Could you check a few things on this model? Use its own coordinates, in mm. Give positions to 0.01 mm unless a question says otherwise; leave off trailing zeros. Order: outer loops, then holes, each group sorted by start corner. A loop starts at its lowest first (then second) coordinate and runs counter-clockwise, first axis right, second up. Notation, with made-up numbers: (50.25, -39) - (97.25, -39) arc R16 ccw to (97.25, -10) - close; hole circle Ø10 at (22, 75.5). An arc over 180 degrees is marked (long way). Put each result on its own line as item: value.
from build123d import *

# Parameters (mm, degrees)
CYLINDER002_R     = 0.3
CYLINDER002_DEPTH = 5
CYLINDER001_R     = 1.3
CYLINDER001_DEPTH = 5
CYLINDER_R        = 6
CYLINDER_DEPTH    = 9.5
CYLINDER003_R     = 0.3
CYLINDER003_DEPTH = 5
FUSION_ROLL_ANGLE = -90


with BuildPart() as obj1:
    # Cylinder002 → Cylinder002 (new body)
    with BuildSketch(Plane(origin=(0, -3.8, -5), x_dir=(1, 0, 0), z_dir=(0, 0, 1))):
        Circle(CYLINDER002_R)
    extrude(amount=CYLINDER002_DEPTH)


with BuildPart() as obj2:
    # Cylinder001 → Cylinder001 (new body)
    with BuildSketch(Plane.XY.offset(4.5)):
        Circle(CYLINDER001_R)
    extrude(amount=CYLINDER001_DEPTH)


with BuildPart() as cut:
    # Cylinder → Cylinder (new body)
    with BuildSketch(Plane.XY):
        Circle(CYLINDER_R)
    extrude(amount=CYLINDER_DEPTH)

    # Cut: cut obj2
    add(obj2.part, mode=Mode.SUBTRACT)


with BuildPart() as buzzer12mm:
    # Cylinder003 → Cylinder003 (new body)
    with BuildSketch(Plane(origin=(0, 3.8, -5), x_dir=(1, 0, 0), z_dir=(0, 0, 1))):
        Circle(CYLINDER003_R)
    extrude(amount=CYLINDER003_DEPTH)

    # Fusion: union obj1, Cut
    add(obj1.part)
    add(cut.part)


with BuildPart() as buzzer12mm_1:
    # Fusion roll: moved
    add(buzzer12mm.part.rotate(Axis((0, 0, 0), (1, 0, 0)), FUSION_ROLL_ANGLE))


with BuildPart() as buzzer12mm_2:
    # Fusion placement: moved
    add(buzzer12mm_1.part.moved(Location((33.37, 5.4, -21.62))))


solid = buzzer12mm_2.part
1) I'm going to push flat-ended pins straight in: pin 1 (5 mm diameter, centred on y = 6.5, z = -26.5, fed in from -X); pin 2 (1.5 mm diameter, centred on x = 35, y = 9.5, fed in from +Z); pin 3 (0.8 mm diameter, centred on x = 34, z = -22, fed in from +Y). Where does each tip first touch, or does it pass through?
Filled in:
pin 1: stops at x = 27.86
pin 2: stops at z = -15.68
pin 3: stops at y = 9.9
2) We'd pull the mould along X, two halves only. Please class faces 1 (the flat face through (33, 9.9, -22)), 2 (the flat face through (35, 14.9, -20)), 3 (the cylindrical face through (28.95, 10.08, -25.68)): pulls with the +X half, pulls with the -X half, needs draft (parallel to the pull), parting line crosses it, or undercut.
Filled in:
face 1: undercut
face 2: needs draft
face 3: parting line crosses it
3) Suppose I cut it at B-B, the plane x = 33.37. List the corners of the cut face in (y, z) for me.
Filled in:
outline: (0.4, -25.72) - (5.4, -25.72) - (5.4, -27.62) - (14.9, -27.62) - (14.9, -22.92) - (9.9, -22.92) - (9.9, -20.32) - (14.9, -20.32) - (14.9, -15.62) - (5.4, -15.62) - (5.4, -17.52) - (0.4, -17.52) - (0.4, -18.12) - (5.4, -18.12) - (5.4, -25.12) - (0.4, -25.12) - close
4) Suppose I cut it at A-A, the plane z = -21.62. List the corners of the cut face in (x, y) for me, and give its area (3 significant figures).
Filled in:
outline: (27.37, 5.4) - (39.37, 5.4) - (39.37, 14.9) - (34.67, 14.9) - (34.67, 9.9) - (32.07, 9.9) - (32.07, 14.9) - (27.37, 14.9) - close
area: 101 mm^2
5) If I drill on line 1 (Z direction, x = 33.37, y = 13); line 2 (X direction, y = 12.9, z = -21.62); line 3 (Z direction, x = 28.5, y = 8.5), over which ranges is the centre line in solid material (lowest first)? Write a range as [from, to].
Filled in:
line 1: z = [-27.62, -22.92], [-20.32, -15.62]
line 2: x = [27.37, 32.07], [34.67, 39.37]
line 3: z = [-25.12, -18.12]
6) Suppose I cut it at D-D, the plane y = 7.75. List the corners of the cut face in (x, z) for me.
Filled in:
outline: circle Ø12 at (33.37, -21.62)
7) Suppose I cut it at C-C, the plane y = 13.25. List the corners of the cut face in (x, z) for me.
Filled in:
outline: circle Ø12 at (33.37, -21.62); hole circle Ø2.6 at (33.37, -21.62)
